```python
from build123d import *

# Parameters (mm, degrees)
SKETCH1_W           = 15
SKETCH1_H           = 74.2
BOSS_EXTRUDE1_DEPTH = 50
SKETCH4_R           = 2.5
CUT_EXTRUDE4_DEPTH  = 4
CHAMFER2_SIZE       = 0.8
SKETCH5_R           = 3.6
CUT_EXTRUDE5_DEPTH  = 15
CHAMFER3_SIZE       = 1.5
SKETCH6_W           = 1.5
SKETCH6_H           = 6
CUT_EXTRUDE6_DEPTH  = 50
SKETCH7_R           = 3.75
CUT_EXTRUDE7_DEPTH  = 5
SKETCH8_R           = 2.05
CUT_EXTRUDE8_DEPTH  = 10


with BuildPart() as part:
    # Sketch1 → Boss-Extrude1 (new body)
    with BuildSketch(Plane.XY):
        with Locations((-7.5, -37.1)):
            Rectangle(SKETCH1_W, SKETCH1_H)
    extrude(amount=BOSS_EXTRUDE1_DEPTH)

    # Sketch4 → Cut-Extrude4 (cut)
    with BuildSketch(Plane.ZY.offset(15)):
        with Locations(Location((43, -25, 0), (0, 0, 270))):
            Circle(SKETCH4_R)
        with Locations(Location((41.217439622, -32.809907304, 0), (0, 0, 270))):
            Circle(SKETCH4_R)
        with Locations(Location((36.222816433, -39.072966684, 0), (0, 0, 270))):
            Circle(SKETCH4_R)
        with Locations(Location((29.005376811, -42.548702419, 0), (0, 0, 270))):
            Circle(SKETCH4_R)
        with Locations(Location((20.994623189, -42.548702419, 0), (0, 0, 270))):
            Circle(SKETCH4_R)
        with Locations(Location((13.777183567, -39.072966684, 0), (0, 0, 270))):
            Circle(SKETCH4_R)
        with Locations(Location((8.782560378, -32.809907304, 0), (0, 0, 270))):
            Circle(SKETCH4_R)
        with Locations(Location((7, -25, 0), (0, 0, 270))):
            Circle(SKETCH4_R)
        with Locations(Location((8.782560378, -17.190092696, 0), (0, 0, 270))):
            Circle(SKETCH4_R)
        with Locations(Location((13.777183567, -10.927033316, 0), (0, 0, 270))):
            Circle(SKETCH4_R)
        with Locations(Location((20.994623189, -7.451297581, 0), (0, 0, 270))):
            Circle(SKETCH4_R)
        with Locations(Location((29.005376811, -7.451297581, 0), (0, 0, 270))):
            Circle(SKETCH4_R)
        with Locations(Location((36.222816433, -10.927033316, 0), (0, 0, 270))):
            Circle(SKETCH4_R)
        with Locations(Location((41.217439622, -17.190092696, 0), (0, 0, 270))):
            Circle(SKETCH4_R)
    extrude(amount=-CUT_EXTRUDE4_DEPTH, mode=Mode.SUBTRACT)

    # Chamfer2
    chamfer2_edges = [part.edges().sort_by_distance(p)[0] for p in [
        (-15, -30.309907304, 41.217439622),
        (-15, -36.572966684, 36.222816433),
        (-15, -40.048702419, 29.005376811),
        (-15, -40.048702419, 20.994623189),
        (-15, -36.572966684, 13.777183567),
        (-15, -30.309907304, 8.782560378),
        (-15, -22.5, 7),
        (-15, -14.690092696, 8.782560378),
        (-15, -8.427033316, 13.777183567),
        (-15, -4.951297581, 20.994623189),
        (-15, -4.951297581, 29.005376811),
        (-15, -8.427033316, 36.222816433),
        (-15, -14.690092696, 41.217439622),
        (-15, -22.5, 43),
    ]]
    chamfer(chamfer2_edges, length=CHAMFER2_SIZE)

    # Sketch5 → Cut-Extrude5 (cut)
    with BuildSketch(Plane.ZY.offset(15)):
        with Locations(Location((25, -25, 0), (0, 0, 270))):
            Circle(SKETCH5_R)
    extrude(amount=-CUT_EXTRUDE5_DEPTH, mode=Mode.SUBTRACT)

    # Chamfer3
    chamfer3_edges = [part.edges().sort_by_distance(p)[0] for p in [
        (-15, -21.4, 25),
    ]]
    chamfer(chamfer3_edges, length=CHAMFER3_SIZE)

    # Sketch6 → Cut-Extrude6 (cut)
    with BuildSketch(Plane.XY.offset(50)):
        with Locations((-0.75, -37.1)):
            Rectangle(SKETCH6_W, SKETCH6_H)
    extrude(amount=-CUT_EXTRUDE6_DEPTH, mode=Mode.SUBTRACT)

    # Sketch7 → Cut-Extrude7 (cut)
    with BuildSketch(Plane.ZY.offset(15)):
        with Locations((15, -64.2)):
            Circle(SKETCH7_R)
        with Locations((35, -64.2)):
            Circle(SKETCH7_R)
        with Locations((5.5, -7.2)):
            Circle(SKETCH7_R)
        with Locations((44.5, -7.2)):
            Circle(SKETCH7_R)
    extrude(amount=-CUT_EXTRUDE7_DEPTH, mode=Mode.SUBTRACT)

    # Sketch8 → Cut-Extrude8 (cut)
    with BuildSketch(Plane.ZY.offset(10)):
        with Locations((35, -64.2)):
            Circle(SKETCH8_R)
        with Locations((15, -64.2)):
            Circle(SKETCH8_R)
        with Locations((5.5, -7.2)):
            Circle(SKETCH8_R)
        with Locations((44.5, -7.2)):
            Circle(SKETCH8_R)
    extrude(amount=-CUT_EXTRUDE8_DEPTH, mode=Mode.SUBTRACT)

    # Chamfer4
    # the kernel refuses this chamfer: 3 mm, written as the material it takes off along each edge
    with BuildSketch(Plane(origin=(-13, -72.2, 48), x_dir=(0.7071067811865476, -0.7071067811865476, 0), z_dir=(-0.5773502691896257, -0.5773502691896257, 0.5773502691896257)), Plane(origin=(-13, -2, 48), x_dir=(0.7071067811865476, 0, 0.7071067811865476), z_dir=(-0.5773502691896257, 0.5773502691896257, 0.5773502691896257))) as chamfer4_piece_1:
        Polygon((-2.121320344, -1.224744871), (2.121320344, -1.224744871), (0, 2.449489743), align=None)
    extrude(amount=3.810511777, mode=Mode.SUBTRACT)
    with BuildSketch(Plane(origin=(-13, -72.2, 2), x_dir=(0.7071067811865476, -0.7071067811865476, 0), z_dir=(-0.5773502691896257, -0.5773502691896257, -0.5773502691896257)), Plane(origin=(-13, -2, 2), x_dir=(0.7071067811865476, 0, -0.7071067811865476), z_dir=(-0.5773502691896257, 0.5773502691896257, -0.5773502691896257))) as chamfer4_piece_2:
        Polygon((-2.121320344, 1.224744871), (2.121320344, 1.224744871), (0, -2.449489743), align=None)
    extrude(amount=3.810511777, mode=Mode.SUBTRACT)
    with BuildSketch(Plane(origin=(7.715048964, -74.2, 50), x_dir=(0, -0.027495876610586768, -0.9996219169112968), z_dir=(-1, 0, 0)), Plane(origin=(-22.715048964, 0, 0), x_dir=(0, -0.9996219169112968, -0.027495876610586372), z_dir=(1, 0, 0))) as chamfer4_piece_3:
        with BuildLine():
            Line((3.086019586, 0), (-0.169641465, -3.081353381))
            Line((-0.169641465, -3.081353381), (-0.22961878, -3.079703628))
            ThreePointArc((-0.22961878, -3.079703628), (-0.102387681, -1.540193489), (-0.059977315, 0.001649753))
            Line((-0.059977315, 0.001649753), (0.001649753, 0.059977315))
            ThreePointArc((0.001649753, 0.059977315), (1.543492994, 0.017566949), (3.087669338, 0.059977315))
            Line((3.087669338, 0.059977315), (3.086019586, 0))
        make_face()
    extrude(amount=30.430097928, mode=Mode.SUBTRACT)
    with BuildSketch(Plane(origin=(-22.715048964, 0, 50), x_dir=(0, -0.9996219169112968, 0.027495876610586778), z_dir=(1, 0, 0)), Plane(origin=(7.715048964, -74.2, 0), x_dir=(0, -0.027495876610586778, 0.9996219169112968), z_dir=(-1, 0, 0))) as chamfer4_piece_4:
        with BuildLine():
            Line((3.086019586, 0), (-0.169641465, 3.081353381))
            Line((-0.169641465, 3.081353381), (-0.22961878, 3.079703628))
            ThreePointArc((-0.22961878, 3.079703628), (-0.102387681, 1.540193489), (-0.059977315, -0.001649753))
            Line((-0.059977315, -0.001649753), (0.001649753, -0.059977315))
            ThreePointArc((0.001649753, -0.059977315), (1.543492994, -0.017566949), (3.087669338, -0.059977315))
            Line((3.087669338, -0.059977315), (3.086019586, 0))
        make_face()
    extrude(amount=30.430097928, mode=Mode.SUBTRACT)
    with BuildSketch(Plane(origin=(-15, -81.915048964, 0), x_dir=(-0.027495876610586202, 0, 0.9996219169112968), z_dir=(0, 1, 0))) as chamfer4_piece_5:
        with BuildLine():
            Line((3.086019586, 0), (-0.169641465, 3.081353381))
            Line((-0.169641465, 3.081353381), (-0.22961878, 3.079703628))
            ThreePointArc((-0.22961878, 3.079703628), (-0.102387681, 1.540193489), (-0.059977315, -0.001649753))
            Line((-0.059977315, -0.001649753), (0.001649753, -0.059977315))
            ThreePointArc((0.001649753, -0.059977315), (1.543492994, -0.017566949), (3.087669338, -0.059977315))
            Line((3.087669338, -0.059977315), (3.086019586, 0))
        make_face()
    extrude(amount=89.630097928, mode=Mode.SUBTRACT)
    with BuildSketch(Plane(origin=(-15, -74.2, -7.715048964), x_dir=(-0.02749587661058619, 0.9996219169112968, 0), z_dir=(0, 0, 1))) as chamfer4_piece_6:
        with BuildLine():
            Line((3.086019586, 0), (-0.169641465, -3.081353381))
            Line((-0.169641465, -3.081353381), (-0.22961878, -3.079703628))
            ThreePointArc((-0.22961878, -3.079703628), (-0.102387681, -1.540193489), (-0.059977315, 0.001649753))
            Line((-0.059977315, 0.001649753), (0.001649753, 0.059977315))
            ThreePointArc((0.001649753, 0.059977315), (1.543492994, 0.017566949), (3.087669338, 0.059977315))
            Line((3.087669338, 0.059977315), (3.086019586, 0))
        make_face()
    extrude(amount=65.430097928, mode=Mode.SUBTRACT)
    with BuildSketch(Plane(origin=(-15, 0, -7.715048964), x_dir=(-0.027495876610586202, -0.9996219169112968, 0), z_dir=(0, 0, 1))) as chamfer4_piece_7:
        with BuildLine():
            Line((3.086019586, 0), (-0.169641465, 3.081353381))
            Line((-0.169641465, 3.081353381), (-0.22961878, 3.079703628))
            ThreePointArc((-0.22961878, 3.079703628), (-0.102387681, 1.540193489), (-0.059977315, -0.001649753))
            Line((-0.059977315, -0.001649753), (0.001649753, -0.059977315))
            ThreePointArc((0.001649753, -0.059977315), (1.543492994, -0.017566949), (3.087669338, -0.059977315))
            Line((3.087669338, -0.059977315), (3.086019586, 0))
        make_face()
    extrude(amount=65.430097928, mode=Mode.SUBTRACT)
    with BuildSketch(Plane(origin=(-15, -81.915048964, 50), x_dir=(-0.02749587661058619, 0, -0.9996219169112968), z_dir=(0, 1, 0))) as chamfer4_piece_8:
        with BuildLine():
            Line((3.086019586, 0), (-0.169641465, -3.081353381))
            Line((-0.169641465, -3.081353381), (-0.22961878, -3.079703628))
            ThreePointArc((-0.22961878, -3.079703628), (-0.102387681, -1.540193489), (-0.059977315, 0.001649753))
            Line((-0.059977315, 0.001649753), (0.001649753, 0.059977315))
            ThreePointArc((0.001649753, 0.059977315), (1.543492994, 0.017566949), (3.087669338, 0.059977315))
            Line((3.087669338, 0.059977315), (3.086019586, 0))
        make_face()
    extrude(amount=89.630097928, mode=Mode.SUBTRACT)


solid = part.part
```
Here's how the part is built. I have some questions about the finished solid (model axes, mm). A direction names the side the tool comes from. Coordinates: 2 decimals unless noted, no trailing zeros. Order: outer loops, then holes, each group sorted by start corner. A loop starts at its lowest first (then second) coordinate and runs counter-clockwise, first axis right, second up.
1) I need wall thicknesses on line 1 (Z direction, x = -12.15, y = -7.2); line 2 (Z direction, x = -11.5, y = -66.5); line 3 (Y direction, x = -7.25, z = 15). Which ranges of each line are inside material? Lowest first, please.
2) Will these pins go through, and if not, where does the flat tip stop? pin 1 (5.5 mm diameter, centred on y = -7.2, z = 5.5, fed in from -X); pin 2 (3 mm diameter, centred on y = -7.45, z = 29.01, fed in from -X); pin 3 (2.5 mm diameter, centred on y = -6, z = 22, fed in from -X).
3) Which directions (+Z, -Z, +X, -X, +Y, -Y) give clear straight access to the entire face, cutting with the end or side of a thin tool? Please do faces 1 (the face through (-6, -37, 50)), 2 (the face through (-12.62, -10.39, 33.78)), 3 (the face through (-1, -40.1, 25)).
4) Imagine slicing it at B-B on x = -9. List the corners of the cut face in (y, z) for me.
5) We'd pull the mould along Y, two halves only. Please class faces 4 (the face through (-6, -2, 1)), 5 (the face through (-12.62, -16.86, 11.26)), 6 (the face through (-14, -38, 2)): +Y half, -Y half, draft (parallel to the pull), parting line (faces both ways), or undercut.
6) Imagine slicing it at A-A on y = -64.2. List the corners of the cut face in (x, z) for me.
7) Imagine slicing it at C-C on y = -25. List the corners of the cut face in (x, z) for me, and give its area (3 significant figures).
Response values:
1. line 1: z = 0.15 to 1.75, 9.25 to 18.51, 23.48 to 26.52, 31.49 to 40.75, 48.25 to 49.85
1. line 2: z = 0 to 12.04, 17.96 to 32.04, 37.96 to 50
1. line 3: y = -74.2 to -66.25, -62.15 to 0
2. pin 1: stops at x = -10
2. pin 2: stops at x = -11
2. pin 3: stops at x = -14.72
3. face 1: +Z, +X, -X, +Y, -Y
3. face 2: -X
3. face 3: +Z, -Z, +X
4. outline: (-74.2, 3) - (-71.2, 0) - (-3, 0) - (0, 3) - (0, 47) - (-3, 50) - (-71.2, 50) - (-74.2, 47) - close; hole circle Ø4.1 at (-64.2, 15); hole circle Ø4.1 at (-64.2, 35); hole circle Ø7.2 at (-25, 25); hole circle Ø4.1 at (-7.2, 5.5); hole circle Ø4.1 at (-7.2, 44.5)
5. face 4: +Y half
5. face 5: undercut
5. face 6: draft
6. outline: (-15, 3) - (-12, 0) - (0, 0) - (0, 12.95) - (-10, 12.95) - (-10, 11.25) - (-15, 11.25) - close; (-15, 18.75) - (-10, 18.75) - (-10, 17.05) - (0, 17.05) - (0, 32.95) - (-10, 32.95) - (-10, 31.25) - (-15, 31.25) - close; (-15, 38.75) - (-10, 38.75) - (-10, 37.05) - (0, 37.05) - (0, 50) - (-12, 50) - (-15, 47) - close
7. outline: (-15, 3) - (-12, 0) - (0, 0) - (0, 21.4) - (-13.5, 21.4) - (-15, 19.9) - (-15, 10.3) - (-14.2, 9.5) - (-11, 9.5) - (-11, 4.5) - (-14.2, 4.5) - (-15, 3.7) - close; (-15, 30.1) - (-13.5, 28.6) - (0, 28.6) - (0, 50) - (-12, 50) - (-15, 47) - (-15, 46.3) - (-14.2, 45.5) - (-11, 45.5) - (-11, 40.5) - (-14.2, 40.5) - (-15, 39.7) - close
7. area: 589 mm2
